The drawing under review shows one solid part. Ordinate dimensions are in mm from its lowest x, y, z. A direction names the side the tool comes from. Give positions to 0.01 mm unless a question says otherwise; leave off trailing zeros. Loops run counter-clockwise (first coordinate to the right, second up) from the corner with the lowest first, then second, coordinate; pieces in that order, holes last. Notation, with made-up numbers: (57, 19) - (71, 19) arc R36 cw to (71, 57) - close; hole circle Ø10 at (-7, 59.5). An arc over 180 degrees is marked (long way). Write each question's results on one line, items separated by ' | '.
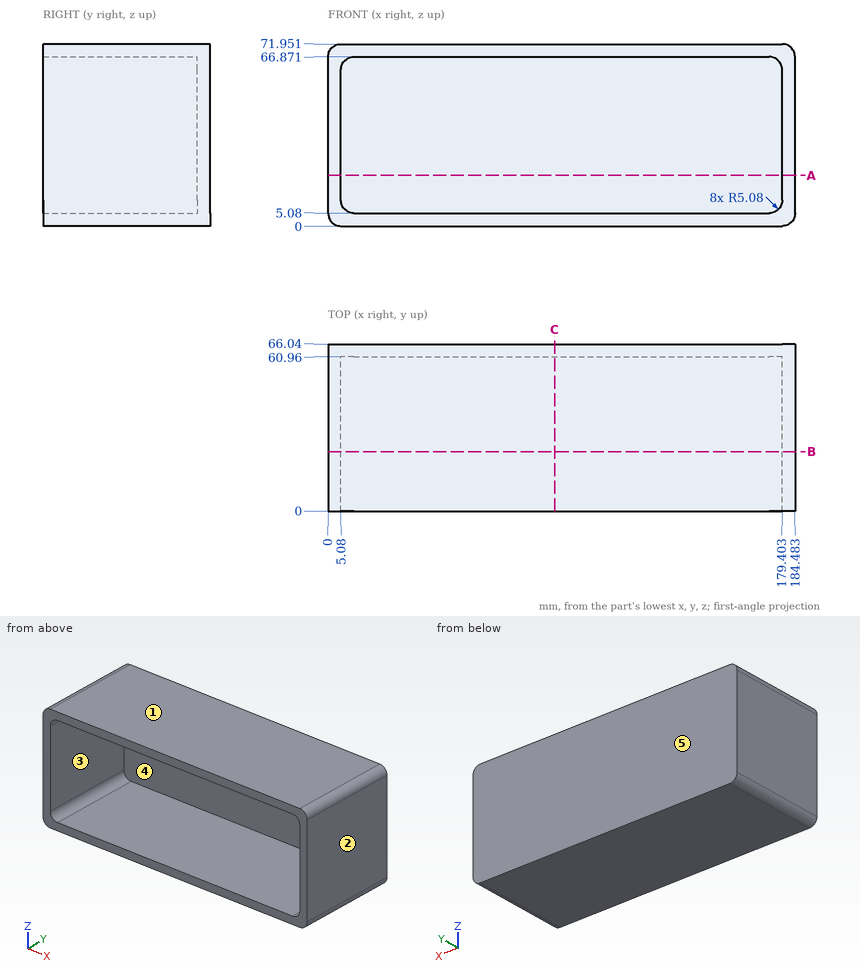
(1) Take a section at A-A on z = 20. Give the boundary of the cut face in (x, y), plus the area to 3 significant figures.
Answers below:
outline: (0, 0) - (5.08, 0) - (5.08, 60.96) - (179.4, 60.96) - (179.4, 0) - (184.48, 0) - (184.48, 66.04) - (0, 66.04) - close | area: 1,560 mm2
(2) Tool access review of the marked faces 4 and 5: name each direction out of +Z, -Z, +X, -X, +Y, -Y from which nothing blocks a thin tool from reaching the whole face with its end or side.
Answers below:
face 4: -Y | face 5: +Z, -Z, +X, -X, +Y
(3) Draft analysis for pull direction X (two halves, no side actions). For the marked faces 1, 2 and 3, state which applies: pulls with the +X half, pulls with the -X half, needs draft (parallel to the pull), parting line crosses it, or undercut.
Answers below:
face 1: needs draft | face 2: pulls with the +X half | face 3: undercut
(4) Take a section at B-B on y = 23.5. Give the boundary of the cut face in (x, z), plus the area to 3 significant figures.
Answers below:
outline: (0, 5.08) arc R5.08 ccw to (5.08, 0) - (179.4, 0) arc R5.08 ccw to (184.48, 5.08) - (184.48, 66.87) arc R5.08 ccw to (179.4, 71.95) - (5.08, 71.95) arc R5.08 ccw to (0, 66.87) - close; hole (5.08, 10.16) arc R5.08 ccw to (10.16, 5.08) - (174.32, 5.08) arc R5.08 ccw to (179.4, 10.16) - (179.4, 61.79) arc R5.08 ccw to (174.32, 66.87) - (10.16, 66.87) arc R5.08 ccw to (5.08, 61.79) - close | area: 2,500 mm2
(5) Take a section at C-C on x = 89.5. Give the boundary of the cut face in (y, z).
Answers below:
outline: (0, 0) - (66.04, 0) - (66.04, 71.95) - (0, 71.95) - (0, 66.87) - (60.96, 66.87) - (60.96, 5.08) - (0, 5.08) - close
(6) Wall thickness on line 1 along Z through (x, y) = (43, 36.5); line 2 along X through (y, z) = (5.5, 53); line 3 along Y through (x, z) = (127, 6): over which ranges is each line inside the solid? List them lowest first. Write a range as from..to.
Answers below:
line 1: 0..5.08, 66.87..71.95 | line 2: 0..5.08, 179.4..184.48 | line 3: 60.96..66.04
(7) Insertion check: P1, Ø3, axis at x = 37, z = 26, coming from the -Y side. The pin has a flat end and moves straight along its axis. Give the tip position at first contact, or say it passes through.
Answers below:
P1: y = 60.96
